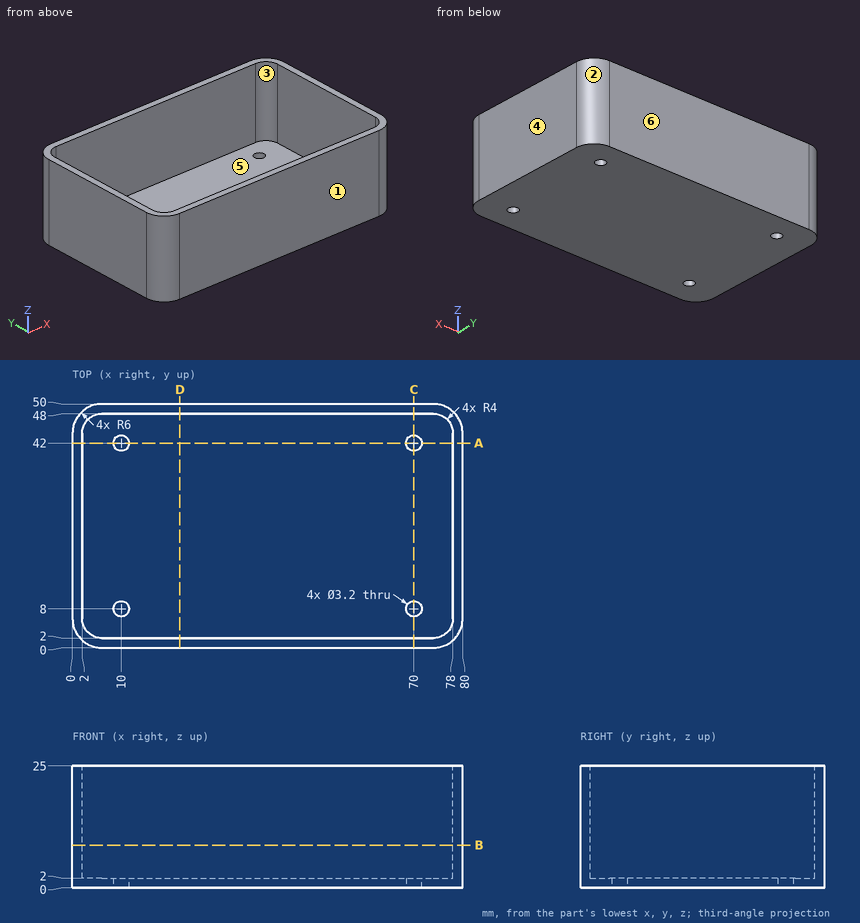
Study the drawing (mm; zero at the part's minimum x, y, z) and answer. A direction names the side the tool comes from. Coordinates: 2 decimals unless noted, no trailing zeros. Write each loop counter-clockwise with the first axis right and the second up, starting at its lowest first coordinate (ties: lowest second). Pieces come first, ordered by that corner, then holes. Notation, with made-up numbers: M 54.25,-31 L 92.25,-31 A35 ccw 92.25,5 Z; hole C -27,-11.75 d8. An arc over 180 degrees is marked long. Use a Markdown table: item, result. Add a question column.
1. Straight lines are drawn through the part: line 1 along Y through (x, z) = (70, 1.45); line 2 along X through (y, z) = (42, 1.1); line 3 along X through (y, z) = (7.5, 8.75). For each, find the intervals that lie inside material, in ascending order. Write a range as [from, to].
2. Section A-A (y = 42) is taken. Give the vertices of the cut face in (x, z), plus the area to 3 significant figures.
3. Which of the six approach directions +Z, -Z, +X, -X, +Y, -Y give full straight-line access (tool end or side, diameter ignored) to the marked faces 5 and 6?
4. Given P1, Ø2, axis at x = 43, y = 26.5, coming from the +Z side; P2, Ø2.5, axis at x = 70, y = 8, coming from the +Z side, each flat-ended and moving along its own axis, determine where each tip first touches the part or whether it passes through.
5. Section C-C (x = 70) is taken. Give the vertices of the cut face in (y, z).
6. For a pull along Y with two mould halves and no side action, classify the marked faces 1, 2, 3 and 4 as +Y half, -Y half, draft (parallel to the pull), parting line (faces both ways), or undercut.
7. Section B-B (z = 8.75) is taken. Give the vertices of the cut face in (x, y), plus the area to 3 significant figures.
8. Section D-D (x = 22) is taken. Give the vertices of the cut face in (y, z), plus the area to 3 significant figures.
Data:
| question | item | result |
|---|---|---|
| 1 | line 1 | y = [0, 6.4], [9.6, 40.4], [43.6, 50] |
| 1 | line 2 | x = [0, 8.4], [11.6, 68.4], [71.6, 80] |
| 1 | line 3 | x = [0, 2], [78, 80] |
| 2 | outline | M 0,0 L 8.4,0 L 8.4,2 L 2,2 L 2,25 L 0,25 Z; M 11.6,0 L 68.4,0 L 68.4,2 L 11.6,2 Z; M 71.6,0 L 80,0 L 80,25 L 78,25 L 78,2 L 71.6,2 Z |
| 2 | area | 239 mm2 |
| 3 | face 5 | +Z |
| 3 | face 6 | +Z, -Z, +X, -X, +Y |
| 4 | P1 | stops at z = 2 |
| 4 | P2 | passes through |
| 5 | outline | M 0,0 L 6.4,0 L 6.4,2 L 2,2 L 2,25 L 0,25 Z; M 9.6,0 L 40.4,0 L 40.4,2 L 9.6,2 Z; M 43.6,0 L 50,0 L 50,25 L 48,25 L 48,2 L 43.6,2 Z |
| 6 | face 1 | -Y half |
| 6 | face 2 | +Y half |
| 6 | face 3 | undercut |
| 6 | face 4 | draft |
| 7 | outline | M 0,6 A6 ccw 6,0 L 74,0 A6 ccw 80,6 L 80,44 A6 ccw 74,50 L 6,50 A6 ccw 0,44 Z; hole M 2,6 A4 ccw 6,2 L 74,2 A4 ccw 78,6 L 78,44 A4 ccw 74,48 L 6,48 A4 ccw 2,44 Z |
| 7 | area | 487 mm2 |
| 8 | outline | M 0,0 L 50,0 L 50,25 L 48,25 L 48,2 L 2,2 L 2,25 L 0,25 Z |
| 8 | area | 192 mm2 |
